Geometry check sheet. Reference: the model listing, model coordinates, mm. Face numbers are marked on the shaded views. A direction names the side the tool comes from. Round coordinates to 2 decimals unless told otherwise and drop trailing zeros. Write each loop counter-clockwise with the first axis right and the second up, starting at its lowest first coordinate (ties: lowest second). Pieces come first, ordered by that corner, then holes. Notation, with made-up numbers: (76.5, -23.75) - (131.5, -23.75) arc R25 ccw to (131.5, -4.75) - close; hole circle Ø2 at (31.25, 39.25). An arc over 180 degrees is marked (long way). Return JSON: item names as keys, results as strings.
```python
from build123d import *

# Parameters (mm, degrees)
BOSS_EXTRUDE1_START = 0.545843
BOSS_EXTRUDE1_DEPTH = 2.445843
FILLET1_R           = 0.257407407


with BuildPart() as part:
    # Sketch2 → Boss-Extrude1 (new body)
    with BuildSketch(Plane(origin=(0, 0, 0), x_dir=(1, 0, 0), z_dir=(0, 1, 0)).offset(BOSS_EXTRUDE1_START)):
        Polygon((2.5, 1.443375673), (0, 2.886751346), (-2.5, 1.443375673), (-2.5, -1.443375673), (0, -2.886751346), (2.5, -1.443375673), align=None)
    extrude(amount=-BOSS_EXTRUDE1_DEPTH)

    # Sketch3 → Cut-Revolve1 (revolve, cut)
    with BuildSketch(Plane.XY):
        Polygon((1.25, 1.267530544), (2.896111111, 0.317147851), (2.896111111, 1.267530544), align=None)
        Polygon((1.25, -2.621687836), (2.896111111, -1.671305143), (2.896111111, -2.621687836), align=None)
    revolve(axis=Axis((0, 1.9, 0), (0, -1, 0)), mode=Mode.SUBTRACT)

    # Fillet1
    fillet1_edges = [part.edges().sort_by_distance(p)[0] for p in [
        (-2.5, -0.677078646, -1.443375673),
        (-2.5, -0.677078646, 1.443375673),
        (0, -0.677078646, 2.886751346),
        (0, -0.677078646, -2.886751346),
        (2.5, -0.677078646, -1.443375673),
        (2.5, -0.677078646, 1.443375673),
    ]]
    fillet(fillet1_edges, radius=FILLET1_R)

    # Sketch5 → Cut-Revolve2 (revolve, cut)
    with BuildSketch(Plane.XY, mode=Mode.PRIVATE) as cut_revolve2_sk:
        Polygon((-1.475, -1.9), (-1.25, -1.675), (-1.25, 0.320842708), (-1.475, 0.545842708), (0, 0.545842708), (0, -1.9), align=None)
    revolve(cut_revolve2_sk.sketch.rotate(Axis((0, 1.9, 0), (0, -1, 0)), 270), axis=Axis((0, 1.9, 0), (0, -1, 0)), mode=Mode.SUBTRACT)


with BuildPart() as revolve1_tool:
    # Sketch4 → Revolve1 (revolve)
    with BuildSketch(Plane.XY):
        with BuildLine():
            Line((-1.475, 1.9), (-2.303125, 1.9))
            ThreePointArc((-2.303125, 1.9), (-2.442336648, 1.842336648), (-2.5, 1.703125))
            Line((-2.5, 1.703125), (-2.5, 0.545842708))
            Line((-2.5, 0.545842708), (-2.4015625, 0.545842708))
            Line((-2.4015625, 0.545842708), (-2.4015625, 1.703125))
            ThreePointArc((-2.4015625, 1.703125), (-2.372730824, 1.772730824), (-2.303125, 1.8015625))
            Line((-2.303125, 1.8015625), (-1.475, 1.8015625))
            Line((-1.475, 1.8015625), (-1.475, 1.9))
        make_face()
    revolve(axis=Axis((0, 1.9, 0), (0, -1, 0)))


with BuildPart() as part_1:
    add(part.part)


with BuildPart() as part_2:
    # Revolve1: joined with revolve1_tool
    add(part_1.part.fuse(revolve1_tool.part, tol=0.00001))


solid = part_2.part
```
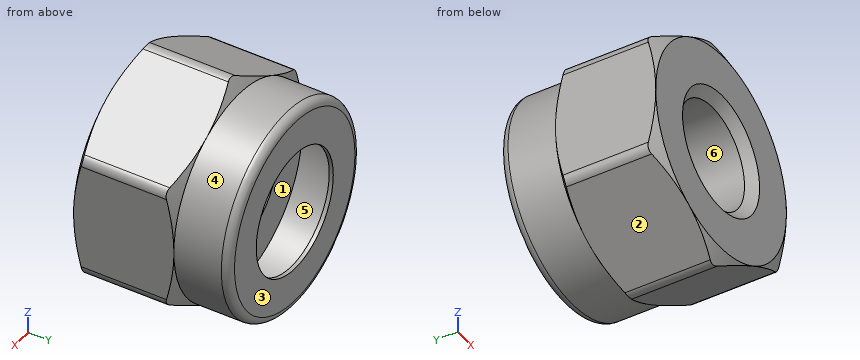
(1) Release check for a two-part mould opening along X. For the marked faces 1, 2 and 3 record: pulls with the +X half, pulls with the -X half, needs draft (parallel to the pull), parting line crosses it, or undercut.
Response values:
{"face 1": "undercut", "face 2": "pulls with the -X half", "face 3": "needs draft"}
(2) Section check B-B, the plane y = -1.05. Enter the section's corners in (x, z), plus the area to 3 significant figures.
Response values:
{"outline": "(-2.5, -1.29) arc R0.26 ccw to (-2.37, -1.52) - (-0.13, -2.81) arc R0.26 ccw to (0.13, -2.81) - (2.37, -1.52) arc R0.26 ccw to (2.5, -1.29) - (2.5, 1.29) arc R0.26 ccw to (2.37, 1.52) - (0.13, 2.81) arc R0.26 ccw to (-0.13, 2.81) - (-2.37, 1.52) arc R0.26 ccw to (-2.5, 1.29) - close; hole circle Ø2.5 at (0, 0)", "area": "16.7 mm^2"}
(3) Section check C-C, the plane y = 1.05. Enter the section's corners in (x, z), plus the area to 3 significant figures.
Response values:
{"outline": "circle Ø5 at (0, 0); hole circle Ø4.8 at (0, 0)", "area": "1.52 mm^2"}
(4) Material ranges on line 1 along X through (y, z) = (-0.25, 0); line 2 along Z through (x, y) = (-2.2, 1.4); line 3 along Z through (x, y) = (-1.1, -1.65), recorded low to high. Write a range as [from, to].
Response values:
{"line 1": "x = [-2.5, -1.25], [1.25, 2.5]", "line 2": "z = [-1.19, -0.96], [0.96, 1.19]", "line 3": "z = [-2.25, -0.59], [0.59, 2.25]"}
(5) Gauge pin test, flat ends, axial feed: pin 1 (1 mm diameter, centred on x = -0.5, y = -1, fed in from -Z); pin 2 (2 mm diameter, centred on x = 0, z = 0, fed in from -Y); pin 3 (1 mm diameter, centred on x = 1, y = 1, fed in from +Z). Record the tip position at first contact, or that the pin passes through.
Response values:
{"pin 1": "stops at z = -2.85", "pin 2": "passes through", "pin 3": "stops at z = 2.45"}
(6) Access from +Z, -Z, +X, -X, +Y, -Y to the whole of each face (thin tool, end or side, straight path). Record for the marked faces 4, 5 and 6.
Response values:
{"face 4": "+Y", "face 5": "none", "face 6": "+Y, -Y"}
